Source: CAD feature listing. Evaluate the final solid. Frame: model axes, mm. A direction names the side the tool comes from. Coordinates: 2 decimals unless noted, no trailing zeros. Order: outer loops, then holes, each group sorted by start corner. A loop starts at its lowest first (then second) coordinate and runs counter-clockwise, first axis right, second up.
```python
from build123d import *

# Parameters (mm, degrees)
SKETCH_1_W          = 10
SKETCH_1_H          = 10
EXTRUDE_1_DEPTH     = 90
SKETCH_2_R          = 2
CUT_EXTRUDE_1_DEPTH = 10
CUT_EXTRUDE_START   = -10
SKETCH_4_R          = 2
CUT_EXTRUDE_2_DEPTH = 10
FILLET_1_R          = 2


with BuildPart() as part:
    # 草图1 → 凸台-拉伸1 (new body)
    with BuildSketch(Plane(origin=(0, 0, 0), x_dir=(1, 0, 0), z_dir=(0, 1, 0))):
        Rectangle(SKETCH_1_W, SKETCH_1_H)
    extrude(amount=EXTRUDE_1_DEPTH)

    # 草图2 → 切除-拉伸1 (cut)
    with BuildSketch(Plane(origin=(0, 90, 0), x_dir=(1, 0, 0), z_dir=(0, 1, 0))):
        with Locations(Location((0, 0, 0), (0, 0, 270))):
            Circle(SKETCH_2_R)
    extrude(amount=-CUT_EXTRUDE_1_DEPTH, mode=Mode.SUBTRACT)

    # 草图4 → 切除-拉伸2 (cut)
    with BuildSketch(Plane.XZ.offset(CUT_EXTRUDE_START)):
        with Locations(Location((0, 0, 0), (0, 0, 90))):
            Circle(SKETCH_4_R)
    extrude(amount=CUT_EXTRUDE_2_DEPTH, mode=Mode.SUBTRACT)

    # 圆角1
    fillet_1_edges = [part.edges().sort_by_distance(p)[0] for p in [
        (-5, 45, -5),
        (5, 45, -5),
        (5, 45, 5),
        (-5, 45, 5),
    ]]
    fillet(fillet_1_edges, radius=FILLET_1_R)


solid = part.part
```
1. Section query B-B on z = 0. Return loops of the section in (x, y), plus the area to 3 significant figures.
Findings:
outline: (-5, 0) - (-2, 0) - (-2, 10) - (2, 10) - (2, 0) - (5, 0) - (5, 90) - (2, 90) - (2, 80) - (-2, 80) - (-2, 90) - (-5, 90) - close
area: 820 mm2
2. Section query C-C on y = 25. Return loops of the section in (x, z), plus the area to 3 significant figures.
Findings:
outline: (-5, -3) arc R2 ccw to (-3, -5) - (3, -5) arc R2 ccw to (5, -3) - (5, 3) arc R2 ccw to (3, 5) - (-3, 5) arc R2 ccw to (-5, 3) - close
area: 96.6 mm2
3. Section query A-A on y = 83. Return loops of the section in (x, z), plus the area to 3 significant figures.
Findings:
outline: (-5, -3) arc R2 ccw to (-3, -5) - (3, -5) arc R2 ccw to (5, -3) - (5, 3) arc R2 ccw to (3, 5) - (-3, 5) arc R2 ccw to (-5, 3) - close; hole circle Ø4 at (0, 0)
area: 84.0 mm2
4. Ray query, line 1 (X direction, y = 6.25, z = 0); line 2 (X direction, y = 59, z = 3.25); line 3 (X direction, y = 8.5, z = 0.5). Return the intervals inside material, ascending.
Findings:
line 1: x = -5 to -2, 2 to 5
line 2: x = -4.98 to 4.98
line 3: x = -5 to -1.94, 1.94 to 5
5. Draft query along Z for faces 1 (the face through (2.2, 90, -0.1)), 2 (the face through (-2, 85, 0)), 3 (the face through (-4.43, 45.63, -4.4)). Return one class per face: released by +Z, released by -Z, zero draft, split by the parting line, or undercut.
Findings:
face 1: zero draft
face 2: undercut
face 3: released by -Z
6. Pin query (flat end, axial travel): P1, Ø1.2, axis at x = 1, z = 0.5, coming from the +Y side; P2, Ø2, axis at x = 0.5, z = 0.5, coming from the -Y side. Return the tip coordinate at first contact, or that it passes through.
Findings:
P1: stops at y = 80
P2: stops at y = 10
7. Access query for faces 4 (the face through (0, 80, 0)), 5 (the face through (2.2, 0, -0.1)), 6 (the face through (2, 5, 0)). Directions: +Z, -Z, +X, -X, +Y, -Y. A direction counts if a zero-diameter tool reaches every point of the face in a straight line with its end or side. Return the directions, or none.
Findings:
face 4: +Y
face 5: +Z, -Z, +X, -X, -Y
face 6: -Y
8. Section query D-D on x = 0. Return loops of the section in (y, z).
Findings:
outline: (0, -5) - (90, -5) - (90, -2) - (80, -2) - (80, 2) - (90, 2) - (90, 5) - (0, 5) - (0, 2) - (10, 2) - (10, -2) - (0, -2) - close
